Here's how the part is built. I have some questions about the finished solid (model axes, mm). A direction names the side the tool comes from. Give positions to 0.01 mm unless a question says otherwise; leave off trailing zeros. Loops run counter-clockwise (first coordinate to the right, second up) from the corner with the lowest first, then second, coordinate; pieces in that order, holes last.
Q1. Suppose I cut it at D-D (x = 50.5). List the corners of the cut face in (y, z) for me.
Q2. For faces 5 (the face through (135, 117, 9)), 6 (the face through (17, 2.3, 9)), which set-ups out of +Z, -Z, +X, -X, +Y, -Y let a thin tool reach every point of the face, with its end or its side?
Q3. Suppose I cut it at A-A (y = 127). List the corners of the cut face in (x, z) for me.
Q4. I need wall thicknesses on probe 1 along X at (y, z) = (122, 12); probe 2 along Y at (x, z) = (31, 6.5); probe 3 along X at (y, z) = (18, 15.25). Which ranges of each line are inside material? Lowest first, please.
Q5. I'm going to push flat-ended pins straight in: P1, Ø9, axis at y = 114.5, z = 12, coming from the -X side; P2, Ø5, axis at y = 16.5, z = 4.5, coming from the -X side; P3, Ø7, axis at y = 107, z = 9, coming from the +X side; P4, Ø9, axis at x = 17.5, z = 5, coming from the +Y side. Where does each tip first touch, or does it pass through?
Q6. Thinking about a two-plate mould opening in Y: for faces 1 (the face through (84, 49, 9)), 2 (the face through (134, 133, 2)), 3 (the face through (133.834, 104.315, 8.404)), 4 (the face through (133.834, 124.315, 8.404)), which applies, pulls with the +Y half, pulls with the -Y half, needs draft (parallel to the pull), parting line crosses it, or undercut?
Q7. Suppose I cut it at B-B (z = 9.75). List the corners of the cut face in (x, y) for me, and give its area (3 significant figures).
Q8. Suppose I cut it at C-C (x = 8). List the corners of the cut face in (y, z) for me, and give its area (4 significant figures).
```python
from build123d import *

# Parameters (mm, degrees)
BOSS_EXTRUDE1_DEPTH = 18
SKETCH2_R           = 2.75
CUT_EXTRUDE1_DEPTH  = 191.153332866
CHAMFER1_SIZE       = 4
SKETCH3_R           = 2.75
CUT_EXTRUDE2_DEPTH  = 192.765481774
CHAMFER2_SIZE       = 4


with BuildPart() as part:
    # Sketch1 → Boss-Extrude1 (new body)
    with BuildSketch(Plane.XY):
        Polygon((0, 0), (35, 0), (135, 100), (135, 135), (132.7, 135), (132.7, 100.952691193), (34.047308807, 2.3), (0, 2.3), align=None)
    extrude(amount=BOSS_EXTRUDE1_DEPTH)

    # Sketch2 → Cut-Extrude1 (cut, through all)
    with BuildSketch(Plane.ZY.offset(-132.7)):
        with Locations((9, 127)):
            Circle(SKETCH2_R)
        with Locations((9, 107)):
            Circle(SKETCH2_R)
    extrude(amount=-CUT_EXTRUDE1_DEPTH, mode=Mode.SUBTRACT)

    # Chamfer1
    chamfer1_edges = [part.edges().sort_by_distance(p)[0] for p in [
        (133.85, 135, 18),
        (133.85, 135, 0),
    ]]
    chamfer(chamfer1_edges, length=CHAMFER1_SIZE)

    # Sketch3 → Cut-Extrude2 (cut, through all)
    with BuildSketch(Plane.XZ):
        with Locations(Location((8, 9, 0), (0, 0, 270))):
            Circle(SKETCH3_R)
        with Locations(Location((28, 9, 0), (0, 0, 270))):
            Circle(SKETCH3_R)
    extrude(amount=-CUT_EXTRUDE2_DEPTH, mode=Mode.SUBTRACT)

    # Chamfer2
    chamfer2_edges = [part.edges().sort_by_distance(p)[0] for p in [
        (0, 1.15, 0),
        (0, 1.15, 18),
    ]]
    chamfer(chamfer2_edges, length=CHAMFER2_SIZE)


solid = part.part
```
Solutions:
1. outline: (15.5, 0) - (18.75, 0) - (18.75, 18) - (15.5, 18) - close
2. face 5: +Z, -Z, +X, +Y, -Y
2. face 6: +Z, -Z, -X, +Y
3. outline: (132.7, 0) - (135, 0) - (135, 6.25) - (132.7, 6.25) - close; (132.7, 11.75) - (135, 11.75) - (135, 18) - (132.7, 18) - close
4. probe 1: x = 132.7 to 135
4. probe 2: y = 0 to 2.3
4. probe 3: x = 49.75 to 53
5. P1: stops at x = 132.7
5. P2: stops at x = 45.75
5. P3: stops at x = 135
5. P4: stops at y = 2.3
6. face 1: pulls with the -Y half
6. face 2: pulls with the +Y half
6. face 3: undercut
6. face 4: undercut
7. outline: (0, 0) - (5.35, 0) - (5.35, 2.3) - (0, 2.3) - close; (10.65, 0) - (25.35, 0) - (25.35, 2.3) - (10.65, 2.3) - close; (30.65, 0) - (35, 0) - (135, 100) - (135, 104.35) - (132.7, 104.35) - (132.7, 100.95) - (34.05, 2.3) - (30.65, 2.3) - close; (132.7, 109.65) - (135, 109.65) - (135, 124.35) - (132.7, 124.35) - close; (132.7, 129.65) - (135, 129.65) - (135, 135) - (132.7, 135) - close
7. area: 433 mm2
8. outline: (0, 0) - (2.3, 0) - (2.3, 6.25) - (0, 6.25) - close; (0, 11.75) - (2.3, 11.75) - (2.3, 18) - (0, 18) - close
8. area: 28.75 mm2
